```python
from build123d import *

# Parameters (mm, degrees)
EXTRUDE_1_DEPTH     = 736
SKETCH_2_W          = 30
SKETCH_2_H          = 16
CUT_EXTRUDE_1_DEPTH = 35


with BuildPart() as part:
    # Эскиз1 → Вытянуть-Тонкостенный1 (new body)
    with BuildSketch(Plane(origin=(0, 0, 0), x_dir=(0, 0, -1), z_dir=(1, 0, 0))):
        Polygon((-10, 15), (-15, 15), (-15, 0), (15, 0), (15, 15), (10, 15), (10, 17), (17, 17), (17, -2), (-17, -2), (-17, 17), (-10, 17), align=None)
    extrude(amount=EXTRUDE_1_DEPTH)

    # Эскиз2 → Вырез-Вытянуть1 (cut, through all)
    with BuildSketch(Plane(origin=(0, 0, -17), x_dir=(-1, 0, 0), z_dir=(0, 0, -1))):
        with Locations((-721, 9)):
            Rectangle(SKETCH_2_W, SKETCH_2_H)
        with Locations((-15, 9)):
            Rectangle(SKETCH_2_W, SKETCH_2_H)
    extrude(amount=-CUT_EXTRUDE_1_DEPTH, mode=Mode.SUBTRACT)


solid = part.part
```
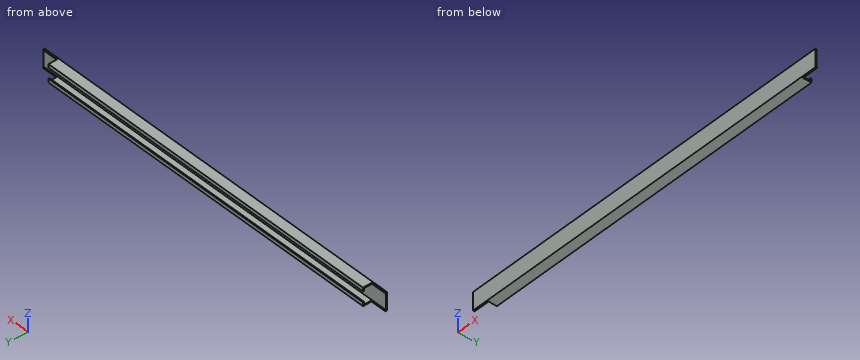
CAD build for the part. Positions are in the model's coordinates, mm. Coordinates: 2 decimals unless noted, no trailing zeros. Order: outer loops, then holes, each group sorted by start corner. A loop starts at its lowest first (then second) coordinate and runs counter-clockwise, first axis right, second up. Notation, with made-up numbers: (-3, 40) - (12, 40) arc R16 ccw to (12, 47) - close; hole circle Ø1 at (-25.5, -11.5). An arc over 180 degrees is marked (long way). Use a Markdown table: item, result. Add a question column.
(1) Saw through at C-C (z = 3). Give the cut face in (x, y), then the cut area to 3 significant figures.
(2) Drill centre lines: line 1 along Z through (x, y) = (677.5, 10); line 2 along Y through (x, z) = (448, -12.5); line 3 along Y through (x, z) = (694.5, 3.5). Where is each one in solid material? Low to high. Write a range as [from, to].
(3) Saw through at B-B (x = 152). Give the cut face in (y, z).
(4) Flat gauge pins, fed straight in: pin 1 (15 mm diameter, centred on x = 306, z = 6, fed in from +Y); pin 2 (7.5 mm diameter, centred on y = 7, z = 15, fed in from -X); pin 3 (2 mm diameter, centred on x = 8, z = 16, fed in from +Y); pin 4 (7.5 mm diameter, centred on y = 11.5, z = -13.5, fed in from +X). Where does each tip first touch, or does it go through?
(5) Saw through at A-A (y = 11.5). Give the cut face in (x, z).
Solved:
| question | item | result |
|---|---|---|
| 1 | outline | (0, -2) - (736, -2) - (736, 0) - (0, 0) - close |
| 1 | area | 1,470 mm² |
| 2 | line 1 | z = [-17, -15], [15, 17] |
| 2 | line 2 | y = [-2, 0], [15, 17] |
| 2 | line 3 | y = [-2, 0] |
| 3 | outline | (-2, -17) - (17, -17) - (17, -10) - (15, -10) - (15, -15) - (0, -15) - (0, 15) - (15, 15) - (15, 10) - (17, 10) - (17, 17) - (-2, 17) - close |
| 4 | pin 1 | stops at y = 17 |
| 4 | pin 2 | stops at x = 30 |
| 4 | pin 3 | stops at y = 1 |
| 4 | pin 4 | stops at x = 706 |
| 5 | outline | (30, -17) - (706, -17) - (706, -15) - (30, -15) - close; (30, 15) - (706, 15) - (706, 17) - (30, 17) - close |
